Design review of the part built by this model. Coordinates are the model's own, in mm. A direction names the side the tool comes from. Give positions to 0.01 mm unless a question says otherwise; leave off trailing zeros. Write each loop counter-clockwise with the first axis right and the second up, starting at its lowest first coordinate (ties: lowest second). Pieces come first, ordered by that corner, then holes. Notation, with made-up numbers: (75.25, 6) -> (119.25, 6) arc R9 cw to (119.25, 22) -> close; hole circle Ø10 at (9, -12.5). An arc over 180 degrees is marked (long way). Write each question's results on one line, items separated by ' | '. Start each with the question number.
(1) To check wall thickness, follow probe 1 along Z at (x, y) = (-41.5, -10); probe 2 along Z at (x, y) = (-37, -5.5); probe 3 along Z at (x, y) = (43.5, -6.75). State the ranges of each line that lie inside material, in increasing order.
(2) Mouldability with a two-part tool opening along X and no side actions: class faces 4 (the face through (-1, 0, 162)), 5 (the face through (-71.485, -7.395, 309.28)), 6 (the face through (-45.43, -7.6, 306.15)) as released by +X, released by -X, zero draft, split by the parting line, or undercut.
(3) Take a section at B-B (z = 263.5). State the section outline as (x, y) points.
(4) Take a section at A-A (x = 65.5). State the section outline as (y, z) points.
(5) For faces 1 (the face through (-53.92, -4.06, 312.97)), 2 (the face through (-49.31, -7.6, 295.63)), 3 (the face through (-75, -7, 155)), list the 3-axis set-ups (+Z, -Z, +X, -X, +Y, -Y) from which the entire face can be reached by the end or side of a thin tool; tool diameter is ignored.
from build123d import *

# Parameters (mm, degrees)
F1_DEPTH = 15
F2_R     = 5
F3_R     = 2
F4_R     = 2
F6_DEPTH = 15.001
F7_R     = 3.1
F8_DEPTH = 9


with BuildPart() as f1:
    # F0 (on Front) → F1 (new body)
    with BuildSketch(Plane.XZ):
        with BuildLine():
            Line((-75, 305.764502), (-75, 0))
            Line((-75, 0), (75, 0))
            Line((75, 0), (75, 245))
            ThreePointArc((75, 245), (33.237011, 312.233185), (-45.541363, 304.590136))
            Line((-45.541363, 304.590136), (-60.857864, 319.906638))
            Line((-60.857864, 319.906638), (-75, 305.764502))
        make_face()
    extrude(amount=F1_DEPTH)

    # F2
    f2_edges = [f1.edges().sort_by_distance(p)[0] for p in [
        (-45.541363, -7.5, 304.590136),
    ]]
    fillet(f2_edges, radius=F2_R)

    # F3
    f3_edges = [f1.edges().sort_by_distance(p)[0] for p in [
        (-60.857864, -7.5, 319.906638),
    ]]
    fillet(f3_edges, radius=F3_R)

    # F4
    f4_edges = [f1.edges().sort_by_distance(p)[0] for p in [
        (-75, -7.5, 305.764502),
    ]]
    fillet(f4_edges, radius=F4_R)

    # F5 (on face) → F6 (cut, through all)
    with BuildSketch(Plane.XZ.offset(15)):
        Polygon((-67.221825, 313.542677), (-68.636039, 312.128463), (-33.308996, 276.80142), (-31.894782, 278.215633), align=None)
    extrude(amount=-F6_DEPTH, mode=Mode.SUBTRACT)

    # F7 (on face) → F8 (cut, through all)
    with BuildSketch(Plane(origin=(129.524387, 0, 129.524387), x_dir=(0.707107, 0, -0.707107), z_dir=(0.707107, 0, 0.707107))):
        with Locations((-259.241161, -7.5)):
            Circle(F7_R)
    extrude(amount=-F8_DEPTH, mode=Mode.SUBTRACT)


solid = f1.part
Report:
1) probe 1: 0 to 284.99, 287.82 to 307.47 | probe 2: 0 to 280.49, 283.32 to 310.24 | probe 3: 0 to 306.1
2) face 4: zero draft | face 5: released by -X | face 6: undercut
3) outline: (-75, -15) -> (72.68, -15) -> (72.68, 0) -> (-75, 0) -> close
4) outline: (-15, 0) -> (0, 0) -> (0, 281.53) -> (-15, 281.53) -> close
5) face 1: +Z, +Y, -Y | face 2: +Y, -Y | face 3: +Z, -Z, -X, +Y, -Y
